Geometry check sheet. Reference: the model listing, model coordinates, mm. A direction names the side the tool comes from. Give positions to 0.01 mm unless a question says otherwise; leave off trailing zeros. Write each loop counter-clockwise with the first axis right and the second up, starting at its lowest first coordinate (ties: lowest second). Pieces come first, ordered by that corner, then holes. Notation, with made-up numbers: (28, -19.75) -> (49, -19.75) arc R20 cw to (49, 11.25) -> close; hole circle Ø2 at (-38, -9.75). An arc over 180 degrees is marked (long way). One line per item, written item: value.
Autodesk Inventor part; units mm, degrees
ref_plane "YZ Plane" through (0, 0, 0) normal (1, 0, 0) x (0, 1, 0)
ref_plane "XZ Plane" through (0, 0, 0) normal (0, 1, 0) x (-1, 0, 0)
ref_plane "XY Plane" through (0, 0, 0) normal (0, 0, 1) x (1, 0, 0)
sketch "Esquisse2" plane through (0, 0, 0) normal (0, 1, 0) x (-1, 0, 0)
  circle A0 centre (0, 0) radius 7.2
  dimension "d0" = 14.4
extrude "Extrusion1" add sketch "Esquisse2" along normal blind 15
sketch "Esquisse4" plane through (0, 15, 0) normal (0, 1, 0) x (1, 0, 0)
  circle A0 centre (0, 0) radius 7.2
  circle A1 centre (0, 0) radius 7.2
  arc A2 (-2, -6.9166) -> (0, -7.2) centre (0, 0) ccw
  arc A3 (-1.4444, -4.9954) -> (0, -5.2) centre (0, 0) ccw
  line L0 (-2, -6.9166) -> (-1.4444, -4.9954)
  line L1 (0, -7.2) -> (0, -5.2)
  line L2 (0, 0) -> (-4.1531, -9.129)
  arc A4 (-5.4277, -4.7308) -> (-3.9, -6.0523) centre (0, 0) ccw
  arc A5 (-3.92, -3.4167) -> (-2.8167, -4.3711) centre (0, 0) ccw
  line L3 (-3.9, -6.0523) -> (-2.8167, -4.3711)
  line L4 (-5.4277, -4.7308) -> (-3.92, -3.4167)
  line L5 (0, -6) -> (0, 5.5969) construction
  line L6 (0, 0) -> (-5.5895, -3.594)
  arc A6 (-6.5507, 2.988) -> (-7.1229, 1.0507) centre (0, 0) ccw
  arc A7 (-4.7311, 2.158) -> (-5.1443, 0.7589) centre (0, 0) ccw
  line L7 (-7.1229, 1.0507) -> (-5.1443, 0.7589)
  line L8 (-6.5507, 2.988) -> (-4.7311, 2.158)
  arc A8 (-7.125, -1.0366) -> (-6.5566, -2.975) centre (0, 0) ccw
  arc A9 (-5.1458, -0.7487) -> (-4.7353, -2.1486) centre (0, 0) ccw
  line L9 (-7.125, -1.0366) -> (-5.1458, -0.7487)
  line L10 (-6.5566, -2.975) -> (-4.7353, -2.1486)
  line L11 (-2, -6.9166) -> (-3.9, -6.0523) construction
  line L12 (-5.4277, -4.7308) -> (-6.5566, -2.975) construction
  line L13 (-2, -6.9166) -> (0, -7.2) construction
  line L14 (0, 0) -> (-5.7368, 3.7048)
  arc A10 (-3.888, 6.06) -> (-5.4183, 4.7415) centre (0, 0) ccw
  line L15 (-5.4183, 4.7415) -> (-3.9132, 3.4244)
  line L16 (-3.888, 6.06) -> (-2.808, 4.3767)
  arc A11 (-2.808, 4.3767) -> (-3.9132, 3.4244) centre (0, 0) ccw
  line L17 (-1.9863, 6.9206) -> (-1.4345, 4.9982)
  arc A12 (0.0143, 7.2) -> (-1.9863, 6.9206) centre (0, 0) ccw
  arc A13 (0.0103, 5.2) -> (-1.4345, 4.9982) centre (0, 0) ccw
  line L18 (0.0143, 7.2) -> (0.0103, 5.2)
  line L19 (-6.5507, 2.988) -> (-5.4183, 4.7415) construction
  line L20 (0, 0) -> (1.7786, 11.975)
  arc A14 (1.9726, -6.9245) -> (3.8184, -6.1041) centre (0, 0) ccw
  arc A15 (1.4246, -5.001) -> (2.7578, -4.4085) centre (0, 0) ccw
  line L21 (1.9726, -6.9245) -> (1.4246, -5.001)
  line L22 (3.8184, -6.1041) -> (2.7578, -4.4085)
  arc A16 (7.1208, -1.0648) -> (7.1364, 0.9551) centre (0, 0) ccw
  line L23 (7.1364, 0.9551) -> (5.154, 0.6898)
  line L24 (7.1208, -1.0648) -> (5.1428, -0.7691)
  arc A17 (5.1428, -0.7691) -> (5.154, 0.6898) centre (0, 0) ccw
  line L25 (6.5161, -3.0627) -> (4.7061, -2.212)
  arc A18 (5.4089, -4.7522) -> (6.5161, -3.0627) centre (0, 0) ccw
  arc A19 (3.9064, -3.4322) -> (4.7061, -2.212) centre (0, 0) ccw
  line L26 (5.4089, -4.7522) -> (3.9064, -3.4322)
  line L27 (3.8184, -6.1041) -> (5.4089, -4.7522) construction
  line L28 (2.079, 6.8933) -> (1.5015, 4.9785)
  arc A20 (2.8253, 4.3655) -> (1.5015, 4.9785) centre (0, 0) ccw
  line L29 (3.912, 6.0445) -> (2.8253, 4.3655)
  arc A21 (3.912, 6.0445) -> (2.079, 6.8933) centre (0, 0) ccw
  arc A22 (4.7396, 2.1392) -> (3.9588, 3.3716) centre (0, 0) ccw
  line L30 (5.4815, 4.6684) -> (3.9588, 3.3716)
  line L31 (6.5625, 2.962) -> (4.7396, 2.1392)
  arc A23 (6.5625, 2.962) -> (5.4815, 4.6684) centre (0, 0) ccw
  line L32 (7.1364, 0.9551) -> (6.5625, 2.962) construction
  line L33 (0.0143, 7.2) -> (2.079, 6.8933) construction
  point P0 (3.8184, -6.1041)
  point P1 (6.5161, -3.0627)
  point P2 (7.1208, -1.0648)
  point P3 (7.1364, 0.9551)
  point P4 (5.4815, 4.6684)
  point P5 (2.079, 6.8933)
  point P6 (-6.5507, 2.988)
  point P7 (-7.1229, 1.0507)
  point P8 (-6.5566, -2.975)
  point P9 (-2, -6.9166)
  point P10 (0, -7.2)
  point P11 (-5.4277, -4.7308)
  point P12 (-3.9, -6.0523)
  dimension "d13" = 2
  dimension "d14" = 2
  dimension "d16" = 1.9
extrude "Extrusion2" cut sketch "Esquisse4" against normal through all contours A0 L24 A17 L23 | L31 A22 L30 A0 | A0 L26 A19 L25 | L29 A20 L28 A0 | A0 L21 A15 L22 | A0 L0 A3 L1 | L18 A13 L17 A0 | L16 A11 L15 A0 | A0 L4 A5 L3 | L8 A7 L7 A0 | A0 L9 A9 L10
sketch "Esquisse5" plane through (0, 15, 0) normal (0, 1, 0) x (1, 0, 0)
  point P0 (0, 0)
sketch "Esquisse6" plane through (0, 15, 0) normal (0, 1, 0) x (1, 0, 0)
  circle A0 centre (0, 0) radius 8
  dimension "d19" = 16
extrude "Extrusion3" add sketch "Esquisse6" along normal blind 1.5
sketch "Esquisse7" plane through (0, 0, 0) normal (0, -1, 0) x (1, 0, 0)
  circle A0 centre (0, 0) radius 8
extrude "Extrusion4" add sketch "Esquisse7" along normal blind 1.5
sketch "Esquisse8" plane through (0, 16.5, 0) normal (0, 1, 0) x (1, 0, 0)
  circle A0 centre (0, 0) radius 4.5
  dimension "d24" = 9
extrude "Extrusion5" cut sketch "Esquisse8" against normal through all
properties part number "Pièce_moteur_courroie_test_2"
1) Sectioned sample at A-A on z = 0. Record the cut outline in (x, y), plus the area to 3 significant figures.
Verdict:
outline: (-8, -1.5) -> (-4.5, -1.5) -> (-4.5, 16.5) -> (-8, 16.5) -> (-8, 15) -> (-7.2, 15) -> (-7.2, 0) -> (-8, 0) -> close; (4.5, -1.5) -> (8, -1.5) -> (8, 0) -> (5.2, 0) -> (5.2, 15) -> (8, 15) -> (8, 16.5) -> (4.5, 16.5) -> close
area: 72.0 mm^2
2) Tool access check on faces 1 (the flat face through (3.38, 7.6, -5.22)), 2 (the flat face through (-3.356, 7.605, -5.23)), 3 (the flat face through (6.159, 7.605, -0.824)). Record the directions out of +Z, -Z, +X, -X, +Y, -Y that give a thin tool (end or side, any length) a straight path to the whole face; none if there is none.
Verdict:
face 1: -Z
face 2: none
face 3: +X
3) Mould release check, pull along Y, two halves, no side actions. Record for faces 4 (the flat face through (3.4, 16.5, 3.4)), 5 (the flat face through (-4.676, 7.605, -4.092)): released by +Y, released by -Y, zero draft, split by the parting line, or undercut.
Verdict:
face 4: released by +Y
face 5: undercut
4) Depth check by flat-ended pin: pin 1 Ø3 at (x, y) = (4, 0.5) entering from -Z; pin 2 Ø4 at (y, z) = (3, 2) entering from +X; pin 3 Ø1 at (y, z) = (5.5, 3) entering from +X. Enter the tip coordinate at first touch or a pass-through.
Verdict:
pin 1: z = -7.57
pin 2: x = 7.12
pin 3: x = 6.75
5) Scan lines: probe 1 along X at (y, z) = (10.75, 0); probe 2 along Y at (x, z) = (6.25, 3.5); probe 3 along X at (y, z) = (12, 2.5). Record each from-to range of solid material in increasing order.
Verdict:
probe 1: -7.2 to -4.5, 4.5 to 5.2
probe 2: -1.5 to 0, 15 to 16.5
probe 3: -5.51 to -3.74, 3.74 to 4.56, 5.32 to 6.75
6) Sectioned sample at B-B on z = 5.75. Record the cut outline in (x, y).
Verdict:
outline: (-5.56, -1.5) -> (5.56, -1.5) -> (5.56, 0) -> (4.33, 0) -> (4.33, 15) -> (5.56, 15) -> (5.56, 16.5) -> (-5.56, 16.5) -> (-5.56, 15) -> (-3.71, 15) -> (-3.71, 0) -> (-5.56, 0) -> close; hole (-1.66, 0) -> (0, 0) -> (0, 15) -> (-1.66, 15) -> close; hole (1.64, 0) -> (3.6, 0) -> (3.6, 15) -> (1.64, 15) -> close
